Autodesk Inventor part; units mm, degrees
ref_plane "YZ Plane" through (0, 0, 0) normal (1, 0, 0) x (0, 1, 0)
ref_plane "XZ Plane" through (0, 0, 0) normal (0, 1, 0) x (-1, 0, 0)
ref_plane "XY Plane" through (0, 0, 0) normal (0, 0, 1) x (1, 0, 0)
sketch "Sketch5" plane through (0, 0, 0) normal (0, 0, 1) x (1, 0, 0)
  line L0 (0, 0) -> (0, 33)
  line L1 (164, 0) -> (164, 33)
  line L2 (164, 33) -> (204, 33)
  line L3 (204, 33) -> (204, 5)
  line L4 (204, 5) -> (209, 5)
  line L5 (209, 5) -> (209, 0)
  line L6 (209, 0) -> (164, 0)
  point P0 (186.5, 0)
  dimension "d16" = 328
  dimension "d17" = 408
  dimension "d19" = 28
  dimension "d20" = 5
  dimension "d21" = 5
revolve "Revolution1" add sketch "Sketch5" angle 360 about axis through (0, 0, 0) along (0, 1, 0)
sketch "Sketch6" plane through (0, 33, 0) normal (0, 1, 0) x (1, 0, 0)
  circle A0 centre (0, 0) radius 184
  line L0 (0, 0) -> (-70.4138, 169.9938)
  line L1 (0, 0) -> (0, 184)
  dimension "d23" = 368
  dimension "d34" = 22.5
hole "Hole1" at (-70.4138, 33, -169.9938) direction (0, -1, 0) diameter 11 end through all counterbore diameter 26 counterbore depth 10
pattern_circular "Circular Pattern2" count 8 over 360 about axis through (0, -10, 0) along (0, 1, 0) of "Hole1"
sketch "Sketch7" plane through (0, 0, 0) normal (0, 1, 0) x (-1, 0, 0)
  circle A0 centre (0, 0) radius 209
  line L0 (0, -209) -> (0, 0)
  line L1 (0, 0) -> (-209, 0)
  circle A1 centre (0, 0) radius 209
extrude "Extrusion5" cut sketch "Sketch7" along normal through all both and the other way through all contours A0 L0 L1 picked at (-105.1818, 91.1406)
equation "\"d29\" = Thickness"
properties part number "DMF 0132 Барабан Опорное кольцо КОРМА четверть"
Could you check a few things on this model? Use its own coordinates, in mm. A direction names the side the tool comes from. Round coordinates to 2 decimals unless told otherwise and drop trailing zeros. Write each loop counter-clockwise with the first axis right and the second up, starting at its lowest first coordinate (ties: lowest second). Pieces come first, ordered by that corner, then holes. Notation, with made-up numbers: M 88.5,86.25 L 134.5,86.25 A18 cw 134.5,105.25 Z; hole C 51,87.5 d2. An arc over 180 degrees is marked long. Write each question's results on one line, items separated by ' | '. Start each with the question number.
1. On a 3-axis mill with a long thin cutter (end or side, diameter ignored), from which of +Z, -Z, +X, -X, +Y, -Y can I reach the whole of each face in a straight line? I mean faces 1 (the face through (164, 23, -71)), 2 (the face through (117.234, 16.731, -114.683)), 3 (the face through (143, 5, -151)). Say none if no direction works.
2. Imagine slicing it at B-B on x = 15.5. List the corners of the cut face in (y, z) for me.
3. Imagine slicing it at C-C on z = -192.5. List the corners of the cut face in (x, y) for me.
4. Imagine slicing it at D-D on y = 13.5. List the corners of the cut face in (x, z) for me, and give its area (3 significant figures).
5. I need wall thicknesses on L1, parallel to X at y = 9, z = -69; L2, parallel to X at y = 25, z = -138; L3, parallel to Z at x = 90, y = 28.5. Which ranges of each line are inside material? Lowest first, please. Write a range as from..to.
6. I'm going to push flat-ended pins straight in: pin 1 Ø17.5 at (x, z) = (70.41, -169.99) entering from -Y; pin 2 Ø2 at (x, y) = (65.5, 12) entering from +Z; pin 3 Ø8 at (x, z) = (168.5, -73) entering from +Y; pin 4 Ø6 at (x, z) = (124.5, -102) entering from -Y. Where does each tip first touch, or does it pass through?
7. Imagine slicing it at A-A on y = 26. List the corners of the cut face in (x, z) for me.
8. Thinking about a two-plate mould opening in Z: for faces 4 (the face through (0, 16, -187)), 5 (the face through (66, 23, -166)), 6 (the face through (164, 27.93, -58.88)), 7 (the face through (186, 16, 0)), which applies, +Z half, -Z half, draft (parallel to the pull), parting line (faces both ways), or undercut?
Result sheet:
1) face 1: +Y | face 2: +Z, -X, +Y, -Y | face 3: -Z, +X, +Y
2) outline: M 0,-208.42 L 5,-208.42 L 5,-203.41 L 33,-203.41 L 33,-163.27 L 0,-163.27 Z
3) outline: M 0,0 L 81.39,0 L 81.39,5 L 67.53,5 L 67.53,33 L 0,33 Z
4) outline: M 0,-204 A204 ccw 204,0 L 164,0 A164 cw 0,-164 Z; hole C 70.41,-169.99 d11; hole C 169.99,-70.41 d11 | area: 11,400 mm^2
5) L1: x = 148.78..164.68, 175.31..191.98 | L2: x = 88.61..150.24 | L3: z = -183.07..-137.1
6) pin 1: stops at y = 0 | pin 2: stops at z = -149.91 | pin 3: stops at y = 23 | pin 4: passes through
7) outline: M 0,-204 A204 ccw 204,0 L 164,0 A164 cw 0,-164 Z; hole C 70.41,-169.99 d26; hole C 169.99,-70.41 d26
8) face 4: draft | face 5: undercut | face 6: undercut | face 7: +Z half
